```python
from build123d import *

# Parameters (mm, degrees)
SKETCH1_R           = 50.8
BOSS_EXTRUDE1_DEPTH = 19.05
CUT_EXTRUDE2_DEPTH  = 15.24
SKETCH5_R           = 4.064
CUT_EXTRUDE3_DEPTH  = 74.440708058
CUT_EXTRUDE4_DEPTH  = 75.324844433
SKETCH7_R           = 48.26
CUT_EXTRUDE5_DEPTH  = 15.24
SKETCH8_R           = 3.2639
CUT_EXTRUDE6_DEPTH  = 74.440708058
CUT_EXTRUDE7_START  = -15.24
SKETCH9_R           = 50.8
CUT_EXTRUDE7_DEPTH  = 15.24
SKETCH10_R          = 6.215985944
BOSS_EXTRUDE2_DEPTH = 3.81


with BuildPart() as part:
    # Sketch1 → Boss-Extrude1 (new body)
    with BuildSketch(Plane(origin=(0, 0, 0), x_dir=(1, 0, 0), z_dir=(0, 1, 0))):
        with Locations(Location((0, 0, 0), (0, 0, 90))):
            Circle(SKETCH1_R)
    extrude(amount=BOSS_EXTRUDE1_DEPTH)

    # Sketch4 → Cut-Extrude2 (cut)
    with BuildSketch(Plane(origin=(0, 19.05, 0), x_dir=(1, 0, 0), z_dir=(0, 1, 0))):
        Polygon((-3.519527241, 6.096), (3.519527241, 6.096), (7.039054482, 0), (3.519527241, -6.096), (-3.519527241, -6.096), (-7.039054482, 0), align=None)
    extrude(amount=-CUT_EXTRUDE2_DEPTH, mode=Mode.SUBTRACT)

    # Sketch5 → Cut-Extrude3 (cut, through all)
    with BuildSketch(Plane(origin=(0, 3.81, 0), x_dir=(1, 0, 0), z_dir=(0, 1, 0))):
        with Locations(Location((0, 0, 0), (0, 0, 270))):
            Circle(SKETCH5_R)
    extrude(amount=-CUT_EXTRUDE3_DEPTH, mode=Mode.SUBTRACT)

    # Sketch6 → Cut-Extrude4 (cut, through all)
    with BuildSketch(Plane(origin=(0, 19.05, 0), x_dir=(1, 0, 0), z_dir=(0, 1, 0))):
        with BuildLine():
            ThreePointArc((-13.470384182, 13.470384182), (-7.290119387, 17.599905094), (0, 19.05))
            Line((0, 19.05), (0, 38.1))
            ThreePointArc((0, 38.1), (-14.580238773, 35.199810189), (-26.940768363, 26.940768363))
            Line((-26.940768363, 26.940768363), (-13.470384182, 13.470384182))
        make_face()
        with BuildLine():
            Line((26.940768363, 26.940768363), (13.470384182, 13.470384182))
            ThreePointArc((13.470384182, 13.470384182), (17.599905094, 7.290119387), (19.05, 0))
            Line((19.05, 0), (38.1, 0))
            ThreePointArc((38.1, 0), (35.199810189, 14.580238773), (26.940768363, 26.940768363))
        make_face()
        with BuildLine():
            Line((26.940768363, -26.940768363), (13.470384182, -13.470384182))
            ThreePointArc((13.470384182, -13.470384182), (7.290119387, -17.599905094), (0, -19.05))
            Line((0, -19.05), (0, -38.1))
            ThreePointArc((0, -38.1), (14.580238773, -35.199810189), (26.940768363, -26.940768363))
        make_face()
        with BuildLine():
            Line((-26.940768363, -26.940768363), (-13.470384182, -13.470384182))
            ThreePointArc((-13.470384182, -13.470384182), (-17.599905094, -7.290119387), (-19.05, 0))
            Line((-19.05, 0), (-38.1, 0))
            ThreePointArc((-38.1, 0), (-35.199810189, -14.580238773), (-26.940768363, -26.940768363))
        make_face()
    extrude(amount=-CUT_EXTRUDE4_DEPTH, mode=Mode.SUBTRACT)

    # Sketch7 → Cut-Extrude5 (cut)
    with BuildSketch(Plane(origin=(0, 19.05, 0), x_dir=(1, 0, 0), z_dir=(0, 1, 0))):
        with Locations(Location((0, 0, 0), (0, 0, 270))):
            Circle(SKETCH7_R)
        with BuildLine():
            Line((-16.313445375, 2.54), (-40.560547334, 2.54))
            ThreePointArc((-40.560547334, 2.54), (-37.546464201, -15.552254691), (-26.884586844, -30.476689292))
            Line((-26.884586844, -30.476689292), (-9.739296625, -13.331399073))
            ThreePointArc((-9.739296625, -13.331399073), (-15.253251082, -6.318103468), (-16.313445375, 2.54))
        make_face(mode=Mode.SUBTRACT)
        with BuildLine():
            Line((16.313445375, -2.54), (40.560547334, -2.54))
            ThreePointArc((40.560547334, -2.54), (37.546464201, 15.552254691), (26.884586844, 30.476689292))
            Line((26.884586844, 30.476689292), (9.739296625, 13.331399073))
            ThreePointArc((9.739296625, 13.331399073), (15.253251082, 6.318103468), (16.313445375, -2.54))
        make_face(mode=Mode.SUBTRACT)
        Polygon((4.985996925, 8.636), (-4.985996925, 8.636), (-9.971993849, 0), (-4.985996925, -8.636), (4.985996925, -8.636), (9.971993849, 0), align=None, mode=Mode.SUBTRACT)
        with BuildLine():
            ThreePointArc((2.54, 40.560547334), (-15.552254691, 37.546464201), (-30.476689292, 26.884586844))
            Line((-30.476689292, 26.884586844), (-13.331399073, 9.739296625))
            ThreePointArc((-13.331399073, 9.739296625), (-6.318103468, 15.253251082), (2.54, 16.313445375))
            Line((2.54, 16.313445375), (2.54, 40.560547334))
        make_face(mode=Mode.SUBTRACT)
        with BuildLine():
            Line((-2.54, -16.313445375), (-2.54, -40.560547334))
            ThreePointArc((-2.54, -40.560547334), (15.552254691, -37.546464201), (30.476689292, -26.884586844))
            Line((30.476689292, -26.884586844), (13.331399073, -9.739296625))
            ThreePointArc((13.331399073, -9.739296625), (6.318103468, -15.253251082), (-2.54, -16.313445375))
        make_face(mode=Mode.SUBTRACT)
    extrude(amount=-CUT_EXTRUDE5_DEPTH, mode=Mode.SUBTRACT)

    # Sketch8 → Cut-Extrude6 (cut, through all)
    with BuildSketch(Plane(origin=(0, 3.81, 0), x_dir=(1, 0, 0), z_dir=(0, 1, 0))):
        with Locations(Location((14.580238773, 35.199810189, 0), (0, 0, 270))):
            Circle(SKETCH8_R)
        with Locations(Location((31.389810189, -10.770238773, 0), (0, 0, 270))):
            Circle(SKETCH8_R)
        with Locations(Location((-14.580238773, -27.579810189, 0), (0, 0, 270))):
            Circle(SKETCH8_R)
        with Locations(Location((-31.389810189, 18.390238773, 0), (0, 0, 270))):
            Circle(SKETCH8_R)
    extrude(amount=-CUT_EXTRUDE6_DEPTH, mode=Mode.SUBTRACT)

    # Sketch9 → Cut-Extrude7 (cut)
    with BuildSketch(Plane(origin=(0, 19.05, 0), x_dir=(1, 0, 0), z_dir=(0, 1, 0)).offset(CUT_EXTRUDE7_START)):
        with Locations(Location((0, 0, 0), (0, 0, 90))):
            Circle(SKETCH9_R)
    extrude(amount=CUT_EXTRUDE7_DEPTH, mode=Mode.SUBTRACT)

    # Sketch10 → Boss-Extrude2 (add)
    with BuildSketch(Plane(origin=(0, 3.81, 0), x_dir=(1, 0, 0), z_dir=(0, 1, 0))):
        Circle(SKETCH10_R)
    extrude(amount=-BOSS_EXTRUDE2_DEPTH)


solid = part.part
```
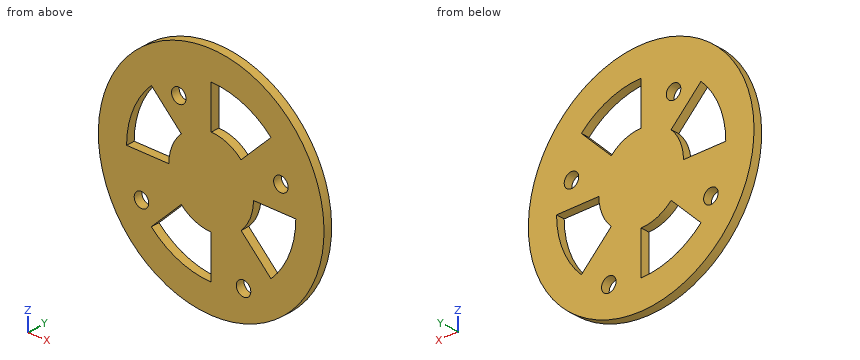
Source: CAD feature listing. Evaluate the final solid. Frame: model axes, mm. Coordinates: 2 decimals unless noted, no trailing zeros. Loops run counter-clockwise (first coordinate to the right, second up) from the corner with the lowest first, then second, coordinate; pieces in that order, holes last. Notation, with made-up numbers: (16, 76.5) -> (65, 76.5) arc R26 ccw to (65, 94.5) -> close; hole circle Ø4 at (62, 69.25). An arc over 180 degrees is marked (long way). One line per item, written item: value. Start each with the question number.
Q1. Section query A-A, the plane x = 33. Return the cut outline in (y, z), and give its area (3 significant figures).
Q2. Contact query for flat-ended pins moving along their axis: P1, Ø1.9, axis at x = 25.5, y = 2.5, coming from the -Z side; P2, Ø1, axis at x = -5, y = 0.5, coming from the -Z side; P3, Ø1.9, axis at y = 1.5, z = -32.5, coming from the -X side. Output: stop coordinate, or through.
Q3. Line query: line 1 along X through (y, z) = (2.25, -26.5); line 2 along Z through (x, y) = (34, 1.4); line 3 along X through (y, z) = (2.85, 16.5). Output: solid intervals per line, ascending.
Q4. Section query C-C, the plane z = 25.5. Return the cut outline in (x, y), and give its area (3 significant figures).
Q5. Section query B-B, the plane z = -7.5. Return the cut outline in (x, y), and give its area (3 significant figures).
Q6. Section query D-D, the plane y = 1.85. Give the number of separate pieces and of enclosed holes in the cut face, and give its area (3 significant figures).
Results:
1. outline: (0, -38.62) -> (3.81, -38.62) -> (3.81, -19.04) -> (0, -19.04) -> close; (0, 0) -> (3.81, 0) -> (3.81, 7.93) -> (0, 7.93) -> close; (0, 13.61) -> (3.81, 13.61) -> (3.81, 38.62) -> (0, 38.62) -> close
1. area: 200 mm^2
2. P1: z = -44.47
2. P2: z = -50.6
2. P3: x = -39.82
3. line 1: -43.34 to -26.5, 0 to 26.5, 27.37 to 43.34
3. line 2: -37.74 to -17.19, 0 to 8.81, 12.73 to 37.74
3. line 3: -48.05 to -34.34, -16.5 to 9.52, 16.5 to 48.05
4. outline: (-43.94, 0) -> (-28.31, 0) -> (-28.31, 3.81) -> (-43.94, 3.81) -> close; (-25.5, 0) -> (-17.1, 0) -> (-17.1, 3.81) -> (-25.5, 3.81) -> close; (-12.06, 0) -> (0, 0) -> (0, 3.81) -> (-12.06, 3.81) -> close; (25.5, 0) -> (43.94, 0) -> (43.94, 3.81) -> (25.5, 3.81) -> close
4. area: 208 mm^2
5. outline: (-50.24, 0) -> (17.51, 0) -> (17.51, 3.81) -> (-50.24, 3.81) -> close; (37.35, 0) -> (50.24, 0) -> (50.24, 3.81) -> (37.35, 3.81) -> close
5. area: 307 mm^2
6. separate pieces: 1
6. enclosed holes: 8
6. area: 6,260 mm^2
